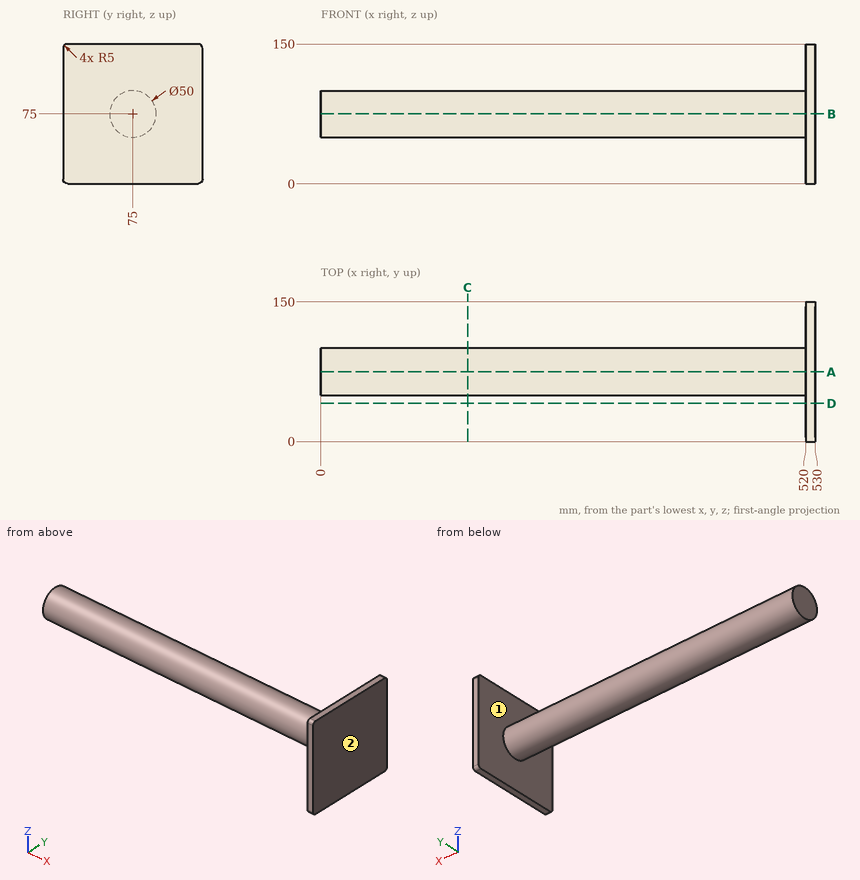
Study the drawing (mm; zero at the part's minimum x, y, z) and answer. A direction names the side the tool comes from. Give positions to 0.01 mm unless a question says otherwise; leave off trailing zeros. Order: outer loops, then holes, each group sorted by start corner. A loop starts at its lowest first (then second) coordinate and runs counter-clockwise, first axis right, second up. Notation, with made-up numbers: (-24.75, 71) - (15.25, 71) arc R17 ccw to (15.25, 83) - close; hole circle Ø1 at (50.25, 44.25). An arc over 180 degrees is marked (long way). Answer as CSV lines item,"result". Start each with the question number.
Q1. The part is cut by section C-C (x = 157.5). Write down the section's boundary in (y, z), then the cut area to 3 significant figures.
Q2. The part is cut by section A-A (y = 75). Write down the section's boundary in (x, z).
Q3. Find the intervals of material crossed by L1, parallel to X at y = 35, z = 112.5; L2, parallel to Y at x = 172.5, z = 76; L3, parallel to Z at x = 256, y = 95.5, in increasing order. Write a range as [from, to].
Q4. Given pin 1 Ø1 at (y, z) = (61, 100.5) entering from -X; pin 2 Ø4 at (x, y) = (283, 56.5) entering from +Z; pin 3 Ø10 at (x, y) = (247, 107) entering from -Z, each flat-ended and moving along its own axis, determine where each tip first touches the part or whether it passes through.
Q5. For the marked faces 1 and 2, determine the directions among +Z, -Z, +X, -X, +Y, -Y from which every point of the face is accessible in a straight line to the end or side of a thin tool.
Q6. The part is cut by section D-D (y = 41). Write down the section's boundary in (x, z).
Check result:
1,outline,"circle Ø50 at (75, 75)"
1,area,"1,960 mm²"
2,outline,"(0, 50) - (520, 50) - (520, 0) - (530, 0) - (530, 150) - (520, 150) - (520, 100) - (0, 100) - close"
3,L1,"x = [520, 530]"
3,L2,"y = [50.02, 99.98]"
3,L3,"z = [60.69, 89.31]"
4,pin 1,"stops at x = 520"
4,pin 2,"stops at z = 93.78"
4,pin 3,"passes through"
5,face 1,"-X"
5,face 2,"+Z, -Z, +X, +Y, -Y"
6,outline,"(520, 0) - (530, 0) - (530, 150) - (520, 150) - close"
